```python
from build123d import *

# Parameters (mm, degrees)
F0_W      = 63.5
F0_H      = 63.5
F1_DEPTH  = 609.6
F2_W      = 254
F2_H      = 101.6
F3_DEPTH  = 12.7
F4_W      = 50.8
F4_H      = 76.2
F5_DEPTH  = 6.35
F6_W      = 6.35
F6_H      = 76.2
F7_DEPTH  = 44.45
F8_W      = 6.35
F8_H      = 76.2
F9_DEPTH  = 44.45
F10_R     = 4.7625
F11_DEPTH = 381


with BuildPart() as f1:
    # F0 (on Top) → F1 (new body)
    with BuildSketch(Plane.XY):
        Polygon((0, 76.2), (0, 0), (76.2, 0), (76.2, 76.2), (6.35, 76.2), (5.991533, 76.2), align=None)
        with Locations((38.1, 38.1)):
            Rectangle(F0_W, F0_H, mode=Mode.SUBTRACT)
    extrude(amount=F1_DEPTH)

    # F2 (on face) → F3 (join)
    with BuildSketch(Plane.XY.offset(609.6)):
        with Locations((38.1, 38.1)):
            Rectangle(F2_W, F2_H)
    extrude(amount=F3_DEPTH)

    # F4 (on face) → F5 (join)
    with BuildSketch(Plane(origin=(0, 0, 609.6), x_dir=(1, 0, 0), z_dir=(0, 0, -1))):
        Polygon((-69.85, 0), (-88.9, 0), (-120.65, 0), (-120.65, -76.2), (-69.85, -76.2), align=None)
        with Locations((171.45, -38.1)):
            Rectangle(F4_W, F4_H)
    extrude(amount=F5_DEPTH)

    # F6 (on face) → F7 (join)
    with BuildSketch(Plane.XY.offset(609.6)):
        with Locations((-117.475, 38.1)):
            Rectangle(F6_W, F6_H)
    extrude(amount=F7_DEPTH)

    # F8 (on face) → F9 (join)
    with BuildSketch(Plane.XY.offset(609.6)):
        with Locations((193.675, 38.1)):
            Rectangle(F8_W, F8_H)
    extrude(amount=F9_DEPTH)

    # F10 (on face) → F11 (cut)
    with BuildSketch(Plane.YZ.offset(196.85)):
        with Locations((19.05, 635)):
            Circle(F10_R)
        with Locations((57.15, 635)):
            Circle(F10_R)
    extrude(amount=-F11_DEPTH, mode=Mode.SUBTRACT)


solid = f1.part
```
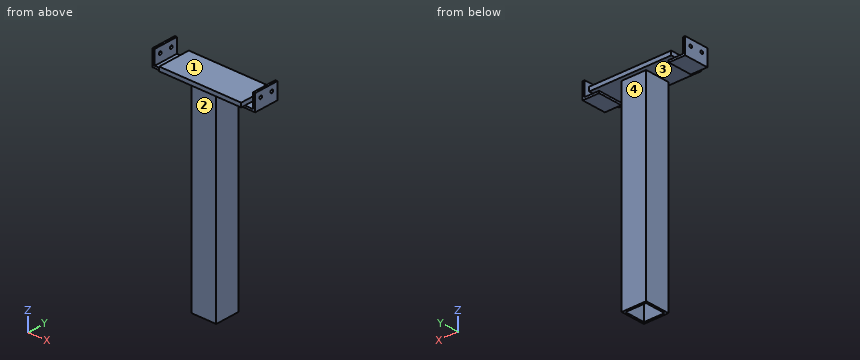
Geometry check sheet. Reference: the model listing, model coordinates, mm. Face numbers are marked on the shaded views. A direction names the side the tool comes from. Round coordinates to 2 decimals unless told otherwise and drop trailing zeros. Loops run counter-clockwise (first coordinate to the right, second up) from the corner with the lowest first, then second, coordinate; pieces in that order, holes last. Notation, with made-up numbers: (15.5, 16.5) - (72.5, 16.5) arc R22 ccw to (72.5, 45.5) - close; hole circle Ø11 at (35, 11). An arc over 180 degrees is marked (long way). Use a Markdown table: item, result.
Q1. Cross-section at C-C on x = 52. Record the cut outline in (y, z).
Solutions:
| item | result |
|---|---|
| outline | (-12.7, 609.6) - (0, 609.6) - (0, 0) - (6.35, 0) - (6.35, 609.6) - (69.85, 609.6) - (69.85, 0) - (76.2, 0) - (76.2, 609.6) - (88.9, 609.6) - (88.9, 622.3) - (-12.7, 622.3) - close |
Q2. Access from +Z, -Z, +X, -X, +Y, -Y to the whole of each face (thin tool, end or side, straight path). Record for the marked faces 1 and 2.
Solutions:
| item | result |
|---|---|
| face 1 | +Z, +Y, -Y |
| face 2 | -Z, +X, -X, -Y |
Q3. Material ranges on line 1 (Y direction, x = 194, z = 635); line 2 (Y direction, x = 16, z = 302), recorded low to high.
Solutions:
| item | result |
|---|---|
| line 1 | y = 0 to 14.29, 23.81 to 52.39, 61.91 to 76.2 |
| line 2 | y = 0 to 6.35, 69.85 to 76.2 |
Q4. Draft check along X on the marked faces 3 and 4. Enter one of: released by +X, released by -X, zero draft, split by the parting line, or undercut.
Solutions:
| item | result |
|---|---|
| face 3 | undercut |
| face 4 | zero draft |
Q5. Go/stop test with flat-tipped pins: P1, Ø1.5, axis at x = 45.5, z = 122, coming from the -Y side; P2, Ø1.5, axis at x = -37.5, y = 70, coming from the -Z side; P3, Ø8, axis at x = 35.5, z = 515.5, coming from the +Y side; P4, Ø8.5, axis at y = 19.05, z = 635, coming from the +X side. Record where each tip stops, or that it passes through.
Solutions:
| item | result |
|---|---|
| P1 | stops at y = 0 |
| P2 | stops at z = 609.6 |
| P3 | stops at y = 76.2 |
| P4 | passes through |
Q6. Cross-section at A-A on z = 381. Record the cut outline in (x, y), plus the area to 3 significant figures.
Solutions:
| item | result |
|---|---|
| outline | (0, 0) - (76.2, 0) - (76.2, 76.2) - (0, 76.2) - close; hole (6.35, 6.35) - (69.85, 6.35) - (69.85, 69.85) - (6.35, 69.85) - close |
| area | 1,770 mm2 |
Q7. Cross-section at B-B on y = 44.5. Record the cut outline in (x, z).
Solutions:
| item | result |
|---|---|
| outline | (-120.65, 603.25) - (-69.85, 603.25) - (-69.85, 609.6) - (0, 609.6) - (0, 0) - (6.35, 0) - (6.35, 609.6) - (69.85, 609.6) - (69.85, 0) - (76.2, 0) - (76.2, 609.6) - (146.05, 609.6) - (146.05, 603.25) - (196.85, 603.25) - (196.85, 654.05) - (190.5, 654.05) - (190.5, 609.6) - (165.1, 609.6) - (165.1, 622.3) - (-88.9, 622.3) - (-88.9, 609.6) - (-114.3, 609.6) - (-114.3, 654.05) - (-120.65, 654.05) - close |
